Source: CAD feature listing. Evaluate the final solid. Frame: model axes, mm. A direction names the side the tool comes from. Round coordinates to 2 decimals unless told otherwise and drop trailing zeros. Order: outer loops, then holes, each group sorted by start corner. A loop starts at its lowest first (then second) coordinate and runs counter-clockwise, first axis right, second up. Notation, with made-up numbers: (75, -7.75) - (90, -7.75) arc R23 ccw to (90, 26.25) - close; hole circle Ø4 at (29, 7). An arc over 180 degrees is marked (long way). Put each result on its own line as item: value. Start each with the question number.
1) Section B-B on y = 2. Output: boundary loops of the cut face in (x, z), then the cut area to 3 significant figures.
2) Section A-A on x = 22.5. Output: boundary loops of the cut face in (y, z).
3) Section C-C on z = 2.5. Output: boundary loops of the cut face in (x, y), then the cut area to 4 significant figures.
4) Line query: probe 1 along X at (y, z) = (-0.75, 11.5); probe 2 along Z at (x, y) = (31.5, 4.75); probe 3 along Z at (x, y) = (4.5, 2.75). Output: solid intervals per line, ascending. Write a range as [from, to].
5) Contact query for flat-ended pins moving along their axis: P1, Ø1.6, axis at x = -4, z = -1.5, coming from the -Y side; P2, Ø4, axis at x = 29.5, y = 6.5, coming from the +Z side; P3, Ø3, axis at y = 7.5, z = 1, coming from the -X side. Output: stop coordinate, or through.
6) Access query for faces 1 (the face through (22, -9, 28)), 2 (the face through (9, -3, 30.778)), 3 (the face through (-4, -3.75, -2)), 4 (the face through (32.497, 7, 28)). Directions: +Z, -Z, +X, -X, +Y, -Y. A direction counts if a zero-diameter tool reaches every point of the face in a straight line with its end or side. Return the directions, or none.
7) Section D-D on x = 10. Output: boundary loops of the cut face in (y, z), then the cut area to 3 significant figures.
Solid Edge part; units mm, degrees
sketch "Sketch1" plane through (0, 0, 0) normal (0, -1, 0) x (1, 0, 0)
  line L0 (38.2914, 27.7776) -> (38.2914, -7.2224)
  line L1 (38.2914, -7.2224) -> (-2.7086, -7.2224)
  line L2 (-2.7086, -7.2224) -> (-2.7086, 27.7776)
  line L3 (-2.7086, 27.7776) -> (38.2914, 27.7776)
  dimension "D1" = 2.7086
  dimension "D2" = 38.2914
extrude "Protrusion1" add sketch "Sketch1" along normal mid plane 19.5
sketch "Sketch2" plane through (17.7914, 0, 27.7776) normal (0, 0, 1) x (1, 0, 0)
  line L0 (-7, 9) -> (14.706, 9)
  line L1 (14.706, 9) -> (14.706, 5.061)
  line L2 (14.706, -5.061) -> (14.706, -9)
  line L3 (14.706, -9) -> (-7, -9)
  arc A0 (-7, -9) -> (-7, 9) centre (-10.75, 0) cw
  arc A1 (14.706, 5.061) -> (14.706, -5.061) centre (11.6575, 0) cw
  dimension "D1" = 14.706
extrude "ProtrusiónExtruida_3" add sketch "Sketch2" along normal blind 1
sketch "Sketch3" plane through (16.3242, 0, 28.7776) normal (0, 0, 1) x (1, 0, 0)
  circle A0 centre (-8.5328, 0) radius 6.5
extrude "ProtrusiónExtruida_4" add sketch "Sketch3" along normal blind 2
sketch "Sketch4" plane through (7.7914, 0, 30.7776) normal (0, 0, 1) x (1, 0, 0)
  circle A0 centre (0, 0) radius 3
extrude "ProtrusiónExtruida_5" add sketch "Sketch4" along normal blind 4
sketch "Sketch5" plane through (-2.7086, 0, 10.2776) normal (-1, 0, 0) x (0, 0, 1)
  line L0 (-14, 3.75) -> (-14, -3.75)
  line L1 (-10, -3.75) -> (-14, -3.75)
  line L2 (-10, 3.75) -> (-10, -3.75)
  line L3 (-14, 3.75) -> (-10, 3.75)
  dimension "D1" = 14
  dimension "D2" = 14
  dimension "D3" = 14
extrude "ProtrusiónExtruida_6" add sketch "Sketch5" along normal blind 2
properties material "Servo"
Answer sheet:
1. outline: (-4.71, -3.72) - (-2.71, -3.72) - (-2.71, -7.22) - (38.29, -7.22) - (38.29, 27.78) - (35.01, 27.78) - (35.01, 28.78) - (13.98, 28.78) - (13.98, 30.78) - (10.03, 30.78) - (10.03, 34.78) - (5.56, 34.78) - (5.56, 30.78) - (1.61, 30.78) - (1.61, 28.78) - (-2.5, 28.78) - (-2.5, 27.78) - (-2.71, 27.78) - (-2.71, 0.28) - (-4.71, 0.28) - close
1. area: 1,520 mm^2
2. outline: (-9.75, -7.22) - (9.75, -7.22) - (9.75, 27.78) - (9, 27.78) - (9, 28.78) - (-9, 28.78) - (-9, 27.78) - (-9.75, 27.78) - close
3. outline: (-2.71, -9.75) - (38.29, -9.75) - (38.29, 9.75) - (-2.71, 9.75) - close
3. area: 799.5 mm^2
4. probe 1: [-2.71, 38.29]
4. probe 2: [-7.22, 28.78]
4. probe 3: [-7.22, 30.78]
5. P1: y = -3.75
5. P2: z = 28.78
5. P3: x = -2.71
6. face 1: +Z, +X, -Y
6. face 2: +Z
6. face 3: +Z, -Z, -X, -Y
6. face 4: +Z, +X, +Y
7. outline: (-9.75, -7.22) - (9.75, -7.22) - (9.75, 27.78) - (9.29, 27.78) - (9.29, 28.78) - (6.11, 28.78) - (6.11, 30.78) - (2.03, 30.78) - (2.03, 34.78) - (-2.03, 34.78) - (-2.03, 30.78) - (-6.11, 30.78) - (-6.11, 28.78) - (-9.29, 28.78) - (-9.29, 27.78) - (-9.75, 27.78) - close
7. area: 742 mm^2
